```python
from build123d import *

# Parameters (mm, degrees)
BOSS_EXTRUDE1_DEPTH        = 10.5
BOSS_EXTRUDE1_2_OUTLINE_W  = 8
BOSS_EXTRUDE1_2_OUTLINE_H  = 5.5
BOSS_EXTRUDE1_START        = -23
BOSS_EXTRUDE1_3_DEPTH      = 2.5
SKETCH2_R                  = 10
BOSS_EXTRUDE2_DEPTH        = 5
BOSS_EXTRUDE3_DEPTH        = 5
SKETCH4_W                  = 11
SKETCH4_H                  = 10
F_12_0_12_DIAMETER_HOLE1_D = 12


with BuildPart() as part:
    # Boss-Extrude1: read off the stored shape, not the designer's step
    # Boss-Extrude1 outline → Boss-Extrude1 (new body)
    with BuildSketch(Plane(origin=(-20.5, 0, 0), x_dir=(0, 0, -1), z_dir=(1, 0, 0))):
        with BuildLine():
            ThreePointArc((-6.184658438, 12), (-6.75, 11.691342951), (-7.299975626, 11.356071321))
            Line((-7.299975626, 11.356071321), (-13.484634065, 0.643928679))
            ThreePointArc((-13.484634065, 0.643928679), (-13.5, 0), (-13.484634065, -0.643928679))
            Line((-13.484634065, -0.643928679), (-7.299975626, -11.356071321))
            ThreePointArc((-7.299975626, -11.356071321), (-6.75, -11.691342951), (-6.184658438, -12))
            Line((-6.184658438, -12), (6.184658438, -12))
            ThreePointArc((6.184658438, -12), (6.75, -11.691342951), (7.299975626, -11.356071321))
            Line((7.299975626, -11.356071321), (13.484634065, -0.643928679))
            ThreePointArc((13.484634065, -0.643928679), (13.5, 0), (13.484634065, 0.643928679))
            Line((13.484634065, 0.643928679), (7.299975626, 11.356071321))
            ThreePointArc((7.299975626, 11.356071321), (6.75, 11.691342951), (6.184658438, 12))
            Line((6.184658438, 12), (-6.184658438, 12))
        make_face()
    extrude(amount=BOSS_EXTRUDE1_DEPTH)

    # Boss-Extrude1 2 outline → Boss-Extrude1 2 (revolve)
    with BuildSketch(Plane.YX):
        with BuildLine():
            ThreePointArc((8, -26), (10.828427125, -24.828427125), (12, -22))
            Line((12, -22), (13.5, -20.5))
            Line((13.5, -20.5), (8, -20.5))
            Line((8, -20.5), (8, -26))
        make_face()
        with Locations((4, -23.25)):
            Rectangle(BOSS_EXTRUDE1_2_OUTLINE_W, BOSS_EXTRUDE1_2_OUTLINE_H)
    revolve(axis=Axis((0, 0, 0), (1, 0, 0)))

    # Boss-Extrude1 3 outline → Boss-Extrude1 3 (cut)
    with BuildSketch(Plane.YZ.offset(BOSS_EXTRUDE1_START)):
        Polygon((0.643928679, 13.484634065), (11.356071321, 7.299975626), (12, 6.92820323), (12, 15), (1.980762112, 15), (0, 13.856406461), align=None)
        Polygon((15, 5.196152422), (12, 6.92820323), (12, -6.92820323), (15, -5.196152422), align=None)
        Polygon((-0.643928679, 13.484634065), (0, 13.856406461), (-1.980762112, 15), (-12, 15), (-12, 6.92820323), (-11.356071321, 7.299975626), align=None)
        Polygon((12, -15), (12, -6.92820323), (11.356071321, -7.299975626), (0.643928679, -13.484634065), (0, -13.856406461), (1.980762112, -15), align=None)
        Polygon((-12, -6.92820323), (-12, 6.92820323), (-15, 5.196152422), (-15, -5.196152422), align=None)
        Polygon((-1.980762112, -15), (0, -13.856406461), (-0.643928679, -13.484634065), (-11.356071321, -7.299975626), (-12, -6.92820323), (-12, -15), align=None)
    extrude(amount=BOSS_EXTRUDE1_3_DEPTH, mode=Mode.SUBTRACT)

    # Sketch2 → Boss-Extrude2 (add)
    with BuildSketch(Plane(origin=(-10, 0, 0), x_dir=(0, 0, -1), z_dir=(1, 0, 0))):
        with Locations(Location((0, 0, 0), (0, 0, 90))):
            Circle(SKETCH2_R)
    extrude(amount=BOSS_EXTRUDE2_DEPTH)

    # Sketch3 → Boss-Extrude3 (add)
    with BuildSketch(Plane(origin=(-5, 0, 0), x_dir=(0, -1, 0), z_dir=(-1, 0, 0))):
        with BuildLine():
            Line((12, -6.184658438), (12, 6.184658438))
            ThreePointArc((12, 6.184658438), (11.691342951, 6.75), (11.356071321, 7.299975626))
            Line((11.356071321, 7.299975626), (0.643928679, 13.484634065))
            ThreePointArc((0.643928679, 13.484634065), (0, 13.5), (-0.643928679, 13.484634065))
            Line((-0.643928679, 13.484634065), (-11.356071321, 7.299975626))
            ThreePointArc((-11.356071321, 7.299975626), (-11.691342951, 6.75), (-12, 6.184658438))
            Line((-12, 6.184658438), (-12, -6.184658438))
            ThreePointArc((-12, -6.184658438), (-11.691342951, -6.75), (-11.356071321, -7.299975626))
            Line((-11.356071321, -7.299975626), (-0.643928679, -13.484634065))
            ThreePointArc((-0.643928679, -13.484634065), (0, -13.5), (0.643928679, -13.484634065))
            Line((0.643928679, -13.484634065), (11.356071321, -7.299975626))
            ThreePointArc((11.356071321, -7.299975626), (11.691342951, -6.75), (12, -6.184658438))
        make_face()
    extrude(amount=-BOSS_EXTRUDE3_DEPTH)

    # Sketch4 → Revolve1 (revolve)
    with BuildSketch(Plane(origin=(0, 0, 0), x_dir=(-1, 0, 0), z_dir=(0, 0, -1)), mode=Mode.PRIVATE) as revolve1_sk:
        with Locations((-5.5, 5)):
            Rectangle(SKETCH4_W, SKETCH4_H)
    revolve(revolve1_sk.sketch.rotate(Axis((11, 0, 0), (-1, 0, 0)), 270), axis=Axis((11, 0, 0), (-1, 0, 0)))

    # Ø12.0 (12) Diameter Hole1 (through all)
    with Locations(Plane.ZY.offset(26)):
        with Locations((0, 0)):
            Hole(F_12_0_12_DIAMETER_HOLE1_D / 2)


solid = part.part
```
Model file for the job. Use its own axes, mm. Give positions to 0.01 mm unless a question says otherwise; leave off trailing zeros. Write each loop counter-clockwise with the first axis right and the second up, starting at its lowest first coordinate (ties: lowest second). Pieces come first, ordered by that corner, then holes. Notation, with made-up numbers: M 55,42 L 94,42 A28 ccw 94,61 Z; hole C -7,43.25 d9. An arc over 180 degrees is marked long. Use a Markdown table: item, result.
1) Cut at B-B (y = 0). List the corners of the cut face in (x, z), and give its area (3 significant figures).
Responses:
| item | result |
|---|---|
| outline | M -26,-8 A4 ccw -22,-12 L -20.5,-13.5 L -10,-13.5 L -10,-10 L -5,-10 L -5,-13.5 L 0,-13.5 L 0,-10 L 11,-10 L 11,-6 L -26,-6 Z; M -26,6 L 11,6 L 11,10 L 0,10 L 0,13.5 L -5,13.5 L -5,10 L -10,10 L -10,13.5 L -20.5,13.5 L -22,12 A4 ccw -26,8 Z |
| area | 422 mm2 |
2) Cut at C-C (x = 3). List the corners of the cut face in (y, z).
Responses:
| item | result |
|---|---|
| outline | C 0,0 d20; hole C 0,0 d12 |
3) Cut at A-A (x = -4). List the corners of the cut face in (y, z).
Responses:
| item | result |
|---|---|
| outline | M -12,-6.18 A13.5 ccw -11.36,-7.3 L -0.64,-13.48 A13.5 ccw 0.64,-13.48 L 11.36,-7.3 A13.5 ccw 12,-6.18 L 12,6.18 A13.5 ccw 11.36,7.3 L 0.64,13.48 A13.5 ccw -0.64,13.48 L -11.36,7.3 A13.5 ccw -12,6.18 Z; hole C 0,0 d12 |
4) Pin check, flat tips, straight feed: pin 1 (1.5 mm diameter, centred on x = 5.5, y = -8, fed in from -Z); pin 2 (1 mm diameter, centred on x = -11, y = 9, fed in from -Z); pin 3 (1.5 mm diameter, centred on x = -8, z = -3.5, fed in from -Y). Stop position of each tip, or through.
Responses:
| item | result |
|---|---|
| pin 1 | stops at z = -6.89 |
| pin 2 | stops at z = -8.95 |
| pin 3 | stops at y = -9.61 |
5) Pull direction X, two halves, no side cores. Call faces 1 (the flat face through (0, 5, 9)), 2 (the flat face through (-10, 5, 9)), 3 (the flat face through (-16.08, 6.07, -10.35)), 4 (the cylindrical face through (-7.54, -2.17, -9.76)): +X half, -X half, draft (parallel to the pull), parting line (faces both ways), or undercut.
Responses:
| item | result |
|---|---|
| face 1 | +X half |
| face 2 | undercut |
| face 3 | draft |
| face 4 | undercut |
6) Drill centre lines: line 1 (Y direction, x = -11.5, z = 0); line 2 (Y direction, x = 6, z = 3.75); line 3 (Z direction, x = -17, y = 3.5). Where is each one in solid material? Low to high. Write a range as from..to.
Responses:
| item | result |
|---|---|
| line 1 | y = -12..-6, 6..12 |
| line 2 | y = -9.27..-4.68, 4.68..9.27 |
| line 3 | z = -11.84..-4.87, 4.87..11.84 |
